CAD build for the part. Positions are in the model's coordinates, mm. A direction names the side the tool comes from. Give positions to 0.01 mm unless a question says otherwise; leave off trailing zeros. Write each loop counter-clockwise with the first axis right and the second up, starting at its lowest first coordinate (ties: lowest second). Pieces come first, ordered by that corner, then holes. Notation, with made-up numbers: (-29.75, 3.25) - (-1.75, 3.25) arc R22 ccw to (-1.75, 12.25) - close; hole circle Ø7 at (34.5, -27.75). An arc over 180 degrees is marked (long way). Write item = value, one per line. Start each with the question number.
```python
from build123d import *

# Parameters (mm, degrees)
SKETCH_1_R      = 10
SKETCH_1_R_2    = 0.6
EXTRUDE_1_DEPTH = 2
SKETCH_2_R      = 1.5
EXTRUDE_2_DEPTH = 3


with BuildPart() as part:
    # 草圖1 → 填料-伸長1 (new body)
    with BuildSketch(Plane.XY):
        Circle(SKETCH_1_R)
        with Locations((4.408389392, 6.067627458)):
            Circle(SKETCH_1_R_2, mode=Mode.SUBTRACT)
        with Locations((0, 7.5)):
            Circle(SKETCH_1_R_2, mode=Mode.SUBTRACT)
        with Locations((7.132923872, 2.317627458)):
            Circle(SKETCH_1_R_2, mode=Mode.SUBTRACT)
        with Locations((7.132923872, -2.317627458)):
            Circle(SKETCH_1_R_2, mode=Mode.SUBTRACT)
        with Locations((4.408389392, -6.067627458)):
            Circle(SKETCH_1_R_2, mode=Mode.SUBTRACT)
        with Locations((0, -7.5)):
            Circle(SKETCH_1_R_2, mode=Mode.SUBTRACT)
        with Locations((-4.408389392, -6.067627458)):
            Circle(SKETCH_1_R_2, mode=Mode.SUBTRACT)
        with Locations((-7.132923872, -2.317627458)):
            Circle(SKETCH_1_R_2, mode=Mode.SUBTRACT)
        with Locations((-7.132923872, 2.317627458)):
            Circle(SKETCH_1_R_2, mode=Mode.SUBTRACT)
        with Locations((-4.408389392, 6.067627458)):
            Circle(SKETCH_1_R_2, mode=Mode.SUBTRACT)
    extrude(amount=EXTRUDE_1_DEPTH)

    # 草圖2 → 填料-伸長2 (add)
    with BuildSketch(Plane(origin=(0, 0, 0), x_dir=(-1, 0, 0), z_dir=(0, 0, -1))):
        with Locations(Location((0, 0, 0), (0, 0, 180))):
            Circle(SKETCH_2_R)
    extrude(amount=EXTRUDE_2_DEPTH)


solid = part.part
```
1. Cut at B-B (y = 0). Give the cut face in (x, z), then the cut area to 3 significant figures.
2. Tool access for faces 1 (the cylindrical face through (3.97, -5.66, 0.99)), 2 (the cylindrical face through (1.43, -0.45, -1.48)): list every direction of +Z, -Z, +X, -X, +Y, -Y with a clear straight run to the whole face (end or side of a thin tool).
3. Cut at C-C (y = -7.75). Give the cut face in (x, z).
4. Mould opens along Y. For faces 3 (the cylindrical face through (-2.17, -9.76, 0.99)), 4 (the flat face through (0, 0, 2)), 5 (the cylindrical face through (-4.85, -5.66, 0.99)) say: +Y half, -Y half, draft (parallel to the pull), parting line (faces both ways), or undercut.
5. Wall check: line 1 along Y through (x, z) = (0, 0.6); line 2 along X through (y, z) = (2.75, 0.3); line 3 along Y through (x, z) = (-7.5, 0.35). Give the ranges that are in metal, low to high.
6. Pin check, flat tip, straight feed: pin 1 Ø1.6 at (x, y) = (-4.41, -6.07) entering from -Z. Stop position of the tip, or through.
7. Cut at D-D (z = 1.25). Count the separate pieces of the cut face and the enclosed holes in it, then the cut area to 3 significant figures.
8. Cut at A-A (x = 0). Give the cut face in (y, z), then the cut area to 3 significant figures.
Output:
q1.outline = (-10, 0) - (-1.5, 0) - (-1.5, -3) - (1.5, -3) - (1.5, 0) - (10, 0) - (10, 2) - (-10, 2) - close
q1.area = 49.0 mm2
q2.face_1 = +Z, -Z
q2.face_2 = -Z
q3.outline = (-6.32, 0) - (-0.55, 0) - (-0.55, 2) - (-6.32, 2) - close; (0.55, 0) - (6.32, 0) - (6.32, 2) - (0.55, 2) - close
q4.face_3 = parting line
q4.face_4 = draft
q4.face_5 = undercut
q5.line_1 = -10 to -8.1, -6.9 to 6.9, 8.1 to 10
q5.line_2 = -9.61 to -7.55, -6.72 to 6.72, 7.55 to 9.61
q5.line_3 = -6.61 to -2.79, -1.84 to 1.84, 2.79 to 6.61
q6.pin_1 = 0
q7.separate_pieces = 1
q7.enclosed_holes = 10
q7.area = 303 mm2
q8.outline = (-10, 0) - (-8.1, 0) - (-8.1, 2) - (-10, 2) - close; (-6.9, 0) - (-1.5, 0) - (-1.5, -3) - (1.5, -3) - (1.5, 0) - (6.9, 0) - (6.9, 2) - (-6.9, 2) - close; (8.1, 0) - (10, 0) - (10, 2) - (8.1, 2) - close
q8.area = 44.2 mm2
